Design review of the part built by this model. Coordinates are the model's own, in mm. Face numbers are marked on the shaded views. A direction names the side the tool comes from. Give positions to 0.01 mm unless a question says otherwise; leave off trailing zeros. Write each loop counter-clockwise with the first axis right and the second up, starting at its lowest first coordinate (ties: lowest second). Pieces come first, ordered by that corner, then holes. Notation, with made-up numbers: (-4, -6.5) - (6, -6.5) arc R19 ccw to (6, -0.5) - close; hole circle Ø3 at (-10, -18.75). An arc over 180 degrees is marked (long way). Write each question's results on one line, items separated by ' | '. Start each with the question number.
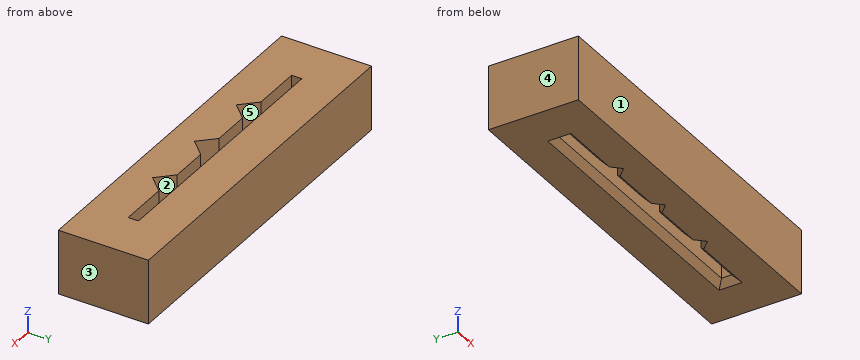
from build123d import *

# Parameters (mm, degrees)
SKETCH_1_W          = 28
SKETCH_1_H          = 7
EXTRUDE_1_DEPTH     = 5
CUT_EXTRUDE_1_DEPTH = 16.272524349
CHAMFER_1_SIZE      = 0.5


with BuildPart() as part:
    # Эскиз1 → Бобышка-Вытянуть1 (new body)
    with BuildSketch(Plane(origin=(0, 66.754264805, 0), x_dir=(-1, 0, 0), z_dir=(0, 0, 1))):
        with Locations((0, 66.754264805)):
            Rectangle(SKETCH_1_W, SKETCH_1_H)
    extrude(amount=EXTRUDE_1_DEPTH)

    # Эскиз4 → Вырез-Вытянуть1 (cut, through all)
    with BuildSketch(Plane(origin=(0, 0, 0), x_dir=(-1, 0, 0), z_dir=(0, 0, -1))):
        Polygon((-10.25, -0.4), (-10.25, 0.4), (10.25, 0.4), (10.25, -0.4), (6.4, -0.4), (5.25, -1.6), (4.1, -0.4), (1.15, -0.4), (0, -1.6), (-1.15, -0.4), (-4.1, -0.4), (-5.25, -1.6), (-6.4, -0.4), align=None)
    extrude(amount=-CUT_EXTRUDE_1_DEPTH, mode=Mode.SUBTRACT)

    # Фаска1
    chamfer_1_edges = [part.edges().sort_by_distance(p)[0] for p in [
        (8.325, -0.4, 0),
        (2.625, -0.4, 0),
        (-2.625, -0.4, 0),
        (-8.325, -0.4, 0),
        (-10.25, 0, 0),
        (0, 0.4, 0),
        (10.25, 0, 0),
    ]]
    chamfer(chamfer_1_edges, length=CHAMFER_1_SIZE)


solid = part.part
Q1. Add section B-B on z = 4.4. State the section outline as (x, y) points.
Q2. For line 1 along Y through (x, z) = (-9.5, 3.8); line 2 along X through (y, z) = (0.25, 2.05); line 3 along Z through (x, y) = (-9, 0.5), list the stretches that pass through material, from the lowest coordinate up. Write a range as [from, to].
Q3. Machinability: for the marked faces 4 and 5, which of the approach directions +Z, -Z, +X, -X, +Y, -Y give a long, thin tool a straight path to every point of the face, cutting with its end or side? Answer none if there is none.
Q4. Add section A-A on x = -3.5. State the section outline as (y, z) points, plus the area to 4 significant figures.
Q5. The part is to be moulded in two halves that separate along Y. For the marked faces 1, 2 and 3, say which applies: +Y half, -Y half, draft (parallel to the pull), parting line (faces both ways), or undercut.
Result:
1) outline: (-14, -3.5) - (14, -3.5) - (14, 3.5) - (-14, 3.5) - close; hole (-10.25, -0.4) - (-6.4, -0.4) - (-5.25, -1.6) - (-4.1, -0.4) - (-1.15, -0.4) - (0, -1.6) - (1.15, -0.4) - (4.1, -0.4) - (5.25, -1.6) - (6.4, -0.4) - (10.25, -0.4) - (10.25, 0.4) - (-10.25, 0.4) - close
2) line 1: y = [-3.5, -0.4], [0.4, 3.5] | line 2: x = [-14, -10.25], [10.25, 14] | line 3: z = [0.4, 5]
3) face 4: +Z, -Z, -X, +Y, -Y | face 5: +Z, -Z
4) outline: (-3.5, 0) - (-0.9, 0) - (-0.4, 0.5) - (-0.4, 5) - (-3.5, 5) - close; (0.4, 0.5) - (0.9, 0) - (3.5, 0) - (3.5, 5) - (0.4, 5) - close | area: 30.75 mm²
5) face 1: -Y half | face 2: undercut | face 3: draft
